Build history of the part. All positions in model axes, mm. A direction names the side the tool comes from. Give positions to 0.01 mm unless a question says otherwise; leave off trailing zeros. Order: outer loops, then holes, each group sorted by start corner. A loop starts at its lowest first (then second) coordinate and runs counter-clockwise, first axis right, second up. Notation, with made-up numbers: (-8.75, 15.5) - (26.25, 15.5) arc R25 cw to (26.25, 52.5) - close; hole circle Ø2 at (37.5, 12.5). An arc over 180 degrees is marked (long way). One line per item, written item: value.
```python
from build123d import *

# Parameters (mm, degrees)
SKETCH_1_R          = 23.5
EXTRUDE_1_DEPTH     = 5
SKETCH_2_R          = 2
CUT_EXTRUDE_1_DEPTH = 59.495923488
SKETCH_3_R          = 12.5
EXTRUDE_3_DEPTH     = 25
SKETCH_4_R          = 4
SKETCH_4_R_2        = 1.5
CUT_EXTRUDE_2_DEPTH = 64.41745079
SKETCH_5_R          = 11
CUT_EXTRUDE_3_DEPTH = 2
CUT_EXTRUDE_START   = -20
SKETCH_6_R          = 2.75
SKETCH_6_R_2        = 1.5
CUT_EXTRUDE_5_DEPTH = 20
EXTRUDE_START       = -23
SKETCH_7_R          = 4
SKETCH_7_R_2        = 2.75
EXTRUDE_4_DEPTH     = 23
FILLET_1_R          = 1


with BuildPart() as part:
    # 草图1 → 凸台-拉伸1 (new body)
    with BuildSketch(Plane.XY):
        with Locations((0, -29.834070393)):
            Circle(SKETCH_1_R)
    extrude(amount=EXTRUDE_1_DEPTH)

    # 草图2 → 切除-拉伸1 (cut, through all)
    with BuildSketch(Plane(origin=(0, 0, 0), x_dir=(-1, 0, 0), z_dir=(0, 0, -1))):
        with Locations((13.699273048, -15.834070393)):
            Circle(SKETCH_2_R)
        with Locations((13.699273048, -43.834070393)):
            Circle(SKETCH_2_R)
        with Locations((-16.800726952, -22.884070393)):
            Circle(SKETCH_2_R)
        with Locations((-16.800726952, -36.884070393)):
            Circle(SKETCH_2_R)
        with Locations((13.699273048, -29.834070393)):
            Circle(SKETCH_2_R)
    extrude(amount=-CUT_EXTRUDE_1_DEPTH, mode=Mode.SUBTRACT)

    # 草图3 → 凸台-拉伸3 (add)
    with BuildSketch(Plane(origin=(0, 0, 0), x_dir=(-1, 0, 0), z_dir=(0, 0, -1))):
        with Locations((0, -29.834070393)):
            Circle(SKETCH_3_R)
    extrude(amount=-EXTRUDE_3_DEPTH)

    # 草图4 → 切除-拉伸2 (cut, through all)
    with BuildSketch(Plane.XY.offset(25)):
        with BuildLine():
            ThreePointArc((-3.5, -24.834070393), (-6.060660172, -23.773410221), (-5, -26.334070393))
            Line((-5, -26.334070393), (-5, -24.834070393))
            Line((-5, -24.834070393), (-3.5, -24.834070393))
        make_face()
        with BuildLine():
            Line((-5, -24.834070393), (-5, -26.334070393))
            ThreePointArc((-5, -26.334070393), (-3.939339828, -25.894730565), (-3.5, -24.834070393))
            Line((-3.5, -24.834070393), (-5, -24.834070393))
        make_face()
        with BuildLine():
            ThreePointArc((3.5, -24.834070393), (3.939339828, -25.894730565), (5, -26.334070393))
            Line((5, -26.334070393), (5, -24.834070393))
            Line((5, -24.834070393), (3.5, -24.834070393))
        make_face()
        with BuildLine():
            Line((5, -24.834070393), (5, -26.334070393))
            ThreePointArc((5, -26.334070393), (6.060660172, -25.894730565), (6.5, -24.834070393))
            ThreePointArc((6.5, -24.834070393), (5, -23.334070393), (3.5, -24.834070393))
            Line((3.5, -24.834070393), (5, -24.834070393))
        make_face()
        with BuildLine():
            ThreePointArc((5, -33.334070393), (3.939339828, -33.773410221), (3.5, -34.834070393))
            Line((3.5, -34.834070393), (5, -34.834070393))
            Line((5, -34.834070393), (5, -33.334070393))
        make_face()
        with BuildLine():
            Line((5, -34.834070393), (3.5, -34.834070393))
            ThreePointArc((3.5, -34.834070393), (5, -36.334070393), (6.5, -34.834070393))
            ThreePointArc((6.5, -34.834070393), (6.060660172, -33.773410221), (5, -33.334070393))
            Line((5, -33.334070393), (5, -34.834070393))
        make_face()
        with Locations((0, -29.834070393)):
            Circle(SKETCH_4_R)
        with Locations((-5, -34.834070393)):
            Circle(SKETCH_4_R_2)
    extrude(amount=-CUT_EXTRUDE_2_DEPTH, mode=Mode.SUBTRACT)

    # 草图5 → 切除-拉伸3 (cut)
    with BuildSketch(Plane.XY.offset(25)):
        with Locations((0, -29.834070393)):
            Circle(SKETCH_5_R)
    extrude(amount=-CUT_EXTRUDE_3_DEPTH, mode=Mode.SUBTRACT)

    # 草图6 → 切除-拉伸5 (cut)
    # profile 1 of 4: a face of its own
    with BuildSketch(Plane(origin=(0, 0, 0), x_dir=(-1, 0, 0), z_dir=(0, 0, -1)).offset(CUT_EXTRUDE_START)):
        with Locations((-5, -24.834070393)):
            Circle(SKETCH_6_R)
        with Locations(Location((-5, -24.834070393, 0), (0, 0, 180))):
            Circle(SKETCH_6_R_2, mode=Mode.SUBTRACT)
    # profile 2 of 4: a face of its own
    with BuildSketch(Plane(origin=(0, 0, 0), x_dir=(-1, 0, 0), z_dir=(0, 0, -1)).offset(CUT_EXTRUDE_START)):
        with Locations((5, -24.834070393)):
            Circle(SKETCH_6_R)
        with Locations(Location((5, -24.834070393, 0), (0, 0, 180))):
            Circle(SKETCH_6_R_2, mode=Mode.SUBTRACT)
    # profile 3 of 4: a face of its own
    with BuildSketch(Plane(origin=(0, 0, 0), x_dir=(-1, 0, 0), z_dir=(0, 0, -1)).offset(CUT_EXTRUDE_START)):
        with Locations((-5, -34.834070393)):
            Circle(SKETCH_6_R)
        with Locations(Location((-5, -34.834070393, 0), (0, 0, 180))):
            Circle(SKETCH_6_R_2, mode=Mode.SUBTRACT)
    # profile 4 of 4: a face of its own
    with BuildSketch(Plane(origin=(0, 0, 0), x_dir=(-1, 0, 0), z_dir=(0, 0, -1)).offset(CUT_EXTRUDE_START)):
        with Locations((5, -34.834070393)):
            Circle(SKETCH_6_R)
        with Locations(Location((5, -34.834070393, 0), (0, 0, 180))):
            Circle(SKETCH_6_R_2, mode=Mode.SUBTRACT)
    extrude(amount=CUT_EXTRUDE_5_DEPTH, mode=Mode.SUBTRACT)

    # 草图7 → 凸台-拉伸4 (add)
    with BuildSketch(Plane(origin=(0, 0, 0), x_dir=(-1, 0, 0), z_dir=(0, 0, -1)).offset(EXTRUDE_START)):
        with Locations((0, -29.834070393)):
            Circle(SKETCH_7_R)
        with Locations((0, -29.834070393)):
            Circle(SKETCH_7_R_2, mode=Mode.SUBTRACT)
    extrude(amount=EXTRUDE_4_DEPTH)

    # 圆角1
    fillet_1_edges = [part.edges().sort_by_distance(p)[0] for p in [
        (12.5, -29.834070393, 5),
    ]]
    fillet(fillet_1_edges, radius=FILLET_1_R)


solid = part.part
```
(1) Slice it at B-B, the plane x = 16. Give the cut face in (y, z), and give its area (3 significant figures).
Completed:
outline: (-47.05, 0) - (-38.72, 0) - (-38.72, 5) - (-47.05, 5) - close; (-35.05, 0) - (-24.72, 0) - (-24.72, 5) - (-35.05, 5) - close; (-21.05, 0) - (-12.62, 0) - (-12.62, 5) - (-21.05, 5) - close
area: 135 mm²
(2) 3-axis set-ups, long thin cutter, end or side, ignore diameter. For faces 4 (the face through (-2, -32, 23)), 5 (the face through (-6.2, -26, 20)), 6 (the face through (-1.478, -27.515, 11.661)): which of +Z, -Z, +X, -X, +Y, -Y reach the whole face in a straight line?
Completed:
face 4: +Z
face 5: -Z
face 6: +Z, -Z
(3) Drill centre lines: line 1 (X direction, y = -30, z = 4.75); line 2 (X direction, y = -22.5, z = 15.5); line 3 (X direction, y = -30, z = 14.25). Where is each one in solid material? Low to high.
Completed:
line 1: -23.5 to -15.69, -12.5 to -2.74, 2.74 to 23.5
line 2: -10.12 to -6.45, -3.55 to 3.55, 6.45 to 10.12
line 3: -12.5 to -2.74, 2.74 to 12.5
(4) Slice it at D-D, the plane y = -48.5. Give the cut face in (x, z).
Completed:
outline: (-14.28, 0) - (14.28, 0) - (14.28, 5) - (-14.28, 5) - close
(5) Slice it at A-A, the plane x = 0. Give the cut face in (y, z).
Completed:
outline: (-53.33, 0) - (-32.58, 0) - (-32.58, 23) - (-40.83, 23) - (-40.83, 25) - (-42.33, 25) - (-42.33, 6) arc R1 cw to (-43.33, 5) - (-53.33, 5) - close; (-27.08, 0) - (-6.33, 0) - (-6.33, 5) - (-16.33, 5) arc R1 cw to (-17.33, 6) - (-17.33, 25) - (-18.83, 25) - (-18.83, 23) - (-27.08, 23) - close
(6) Pull direction X, two halves, no side cores. Call faces 1 (the face through (-15.7, -29.9, 2.3)), 2 (the face through (0, -35, 0)), 3 (the face through (-3.059, -6.534, 2.465)): +X half, -X half, draft (parallel to the pull), parting line (faces both ways), or undercut.
Completed:
face 1: undercut
face 2: draft
face 3: parting line
(7) Pin check, flat tips, straight feed: P1, Ø20, axis at x = 0, y = -29.83, coming from the -Z side; P2, Ø6.5, axis at x = -5, y = -24.83, coming from the +Z side; P3, Ø3, axis at x = -13.7, y = -15.83, coming from the +Z side; P4, Ø3.5, axis at x = -5, y = -34.83, coming from the -Z side. Stop position of each tip, or through.
Completed:
P1: z = 0
P2: z = 23
P3: through
P4: z = 20
(8) Slice it at C-C, the plane z = 11.75. Give the cut face in (x, y).
Completed:
outline: circle Ø25 at (0, -29.83); hole circle Ø5.5 at (-5, -34.83); hole circle Ø5.5 at (-5, -24.83); hole circle Ø5.5 at (0, -29.83); hole circle Ø5.5 at (5, -34.83); hole circle Ø5.5 at (5, -24.83)
